```python
from build123d import *

# Parameters (mm, degrees)
BOSS_EXTRUDE4_DEPTH = 2.5
SKETCH3_W           = 2.85
SKETCH3_H           = 2.5
CUT_EXTRUDE1_DEPTH  = 10
SKETCH4_W           = 2.85
SKETCH4_H           = 2.5
CUT_EXTRUDE2_DEPTH  = 7.5


with BuildPart() as part:
    # Sketch2 → Boss-Extrude4 (new body)
    with BuildSketch(Plane(origin=(0, 0, 0), x_dir=(1, 0, 0), z_dir=(0, 1, 0))):
        Polygon((0, 0), (0.589412548, 2.381206373), (1.144861346, 4.62520037), (1.144861346, 9.49123355), (1.827568156, 12.249345527), (3.377711093, 13.184348171), (5.118763194, 17.917932427), (8.800884637, 20.138884573), (11.280786748, 22.394616205), (14.440798826, 23.447953565), (16.304846177, 24.572294527), (21.3928254, 25.291293944), (26.027509782, 25.291293944), (31.203392004, 24.010124046), (33.156993004, 23.526555316), (34.802606354, 22.921284885), (38.501454152, 23.073163176), (40.508590996, 23.727616723), (41.385127416, 24.256318851), (42.088080237, 27.096224014), (42.502286902, 27.510430679), (42.564029409, 29.84745559), (43.246427291, 31.702763579), (44.023704459, 32.719500007), (45.070889284, 32.719500007), (45.859589446, 32.116552566), (46.507843196, 30.50318738), (47.03069527, 29.201920191), (48.220652238, 28.011963224), (48.608289607, 27.624325855), (49.727600372, 27.510430679), (51.646333081, 26.804704651), (52.922878944, 26.335180347), (54.158394758, 26.335180347), (54.935057216, 26.647245064), (56.282727814, 27.252145785), (57.423923636, 28.011963224), (58.445785658, 28.559225004), (59.674350615, 28.609671077), (60.194070138, 28.212354617), (60.2647419, 26.491212706), (59.967729771, 25.291293944), (59.894673222, 24.256318851), (58.99338734, 22.921284885), (57.847567942, 21.224034494), (57.087511308, 20.098197019), (57.087511308, 16.074592048), (56.063262547, 14.557418737), (55.70254482, 14.023103901), (55.136298029, 13.184348171), (54.820686328, 12.716846849), (53.217353691, 11.749761674), (52.573042644, 9.998004432), (51.646333081, 9.439039274), (51.144861346, 8.07563452), (50.17002425, 6.631652471), (49.432034292, 4.62520037), (49.01935436, 3.503203372), (44.218024527, 0), align=None)
    extrude(amount=BOSS_EXTRUDE4_DEPTH)

    # Sketch3 → Cut-Extrude1 (cut)
    with BuildSketch(Plane.XY):
        with Locations((11.675, 1.25)):
            Rectangle(SKETCH3_W, SKETCH3_H)
    extrude(amount=-CUT_EXTRUDE1_DEPTH, mode=Mode.SUBTRACT)

    # Sketch4 → Cut-Extrude2 (cut)
    with BuildSketch(Plane.XY):
        with Locations((35.793024527, 1.25)):
            Rectangle(SKETCH4_W, SKETCH4_H)
    extrude(amount=-CUT_EXTRUDE2_DEPTH, mode=Mode.SUBTRACT)


solid = part.part
```
Build history of the part. All positions in model axes, mm. A direction names the side the tool comes from. Coordinates: 2 decimals unless noted, no trailing zeros. Order: outer loops, then holes, each group sorted by start corner. A loop starts at its lowest first (then second) coordinate and runs counter-clockwise, first axis right, second up. Notation, with made-up numbers: (33.25, 1.25) -> (47.25, 1.25) arc R22 ccw to (47.25, 26.25) -> close; hole circle Ø10 at (20.25, 68). An arc over 180 degrees is marked (long way). Answer in a Markdown table with one row per item. Add a question column.
Q1. Which spindle directions (+Z, -Z, +X, -X, +Y, -Y) get a long thin tool onto all of the face, cutting with end or side? Do faces 1 (the face through (12, 1, -10)), 2 (the face through (24, 1, -25.291)), 3 (the face through (39.5, 1.2, -23.4)). Say none if no direction does.
Q2. Mould opens along X. For faces 4 (the face through (37.218, 1, -4)), 5 (the face through (42.9, 1.23, -30.76)), 6 (the face through (52.9, 1.23, -10.89)), 7 (the face through (13.1, 1, -5)) say: +X half, -X half, draft (parallel to the pull), parting line (faces both ways), or undercut.
Q3. Band-saw the part on B-B, the plane x = 19. List the corners of the cut face in (y, z).
Q4. Wall check: line 1 along X through (y, z) = (0.25, -28.5); line 2 along X through (y, z) = (0.3, -3); line 3 along X through (y, z) = (1.2, -4). Give the ranges that are in metal, low to high. Write a range as [from, to].
Q5. Band-saw the part on A-A, the plane x = 7. List the corners of the cut face in (y, z).
Q6. Drop flat-ended pins along their axis: pin 1 (1.2 mm diameter, centred on y = 1, z = -2.5, fed in from -X); pin 2 (1.2 mm diameter, centred on y = 1.5, z = -4.5, fed in from +X); pin 3 (1 mm diameter, centred on y = 0.5, z = -7, fed in from -X). Give the stop position or say it passes through.
Answers follow:
| question | item | result |
|---|---|---|
| 1 | face 1 | +Z, +Y, -Y |
| 1 | face 2 | -Z, -X, +Y, -Y |
| 1 | face 3 | -Z, +Y, -Y |
| 2 | face 4 | undercut |
| 2 | face 5 | -X half |
| 2 | face 6 | +X half |
| 2 | face 7 | undercut |
| 3 | outline | (0, -24.95) -> (2.5, -24.95) -> (2.5, 0) -> (0, 0) -> close |
| 4 | line 1 | [42.53, 47.73], [58.34, 59.82] |
| 4 | line 2 | [0.74, 10.25], [13.1, 34.37], [37.22, 48.33] |
| 4 | line 3 | [0.99, 10.25], [13.1, 34.37], [37.22, 49.2] |
| 5 | outline | (0, -19.05) -> (2.5, -19.05) -> (2.5, 0) -> (0, 0) -> close |
| 6 | pin 1 | x = 0.47 |
| 6 | pin 2 | x = 49.61 |
| 6 | pin 3 | x = 1.14 |
